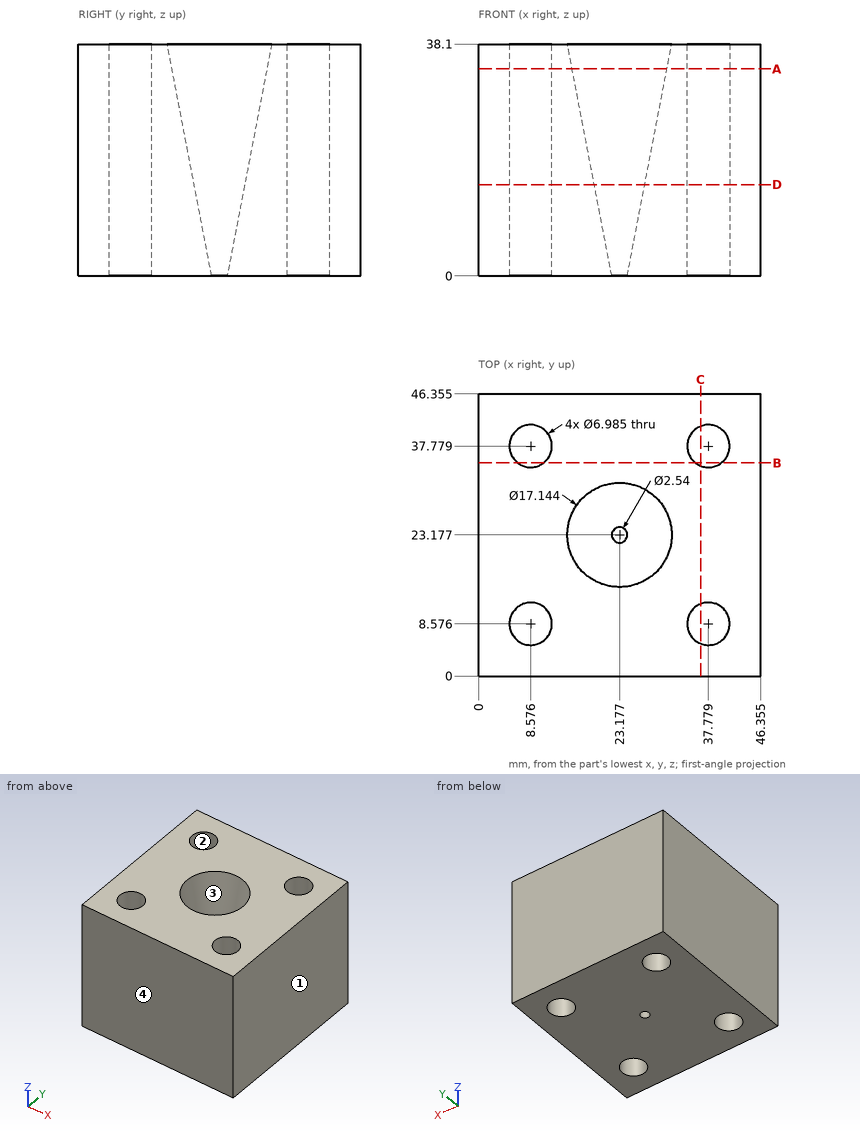
Here's the drawing with two shaded views (mm, measured from the low corner). I have some questions. Round coordinates to 2 decimals unless told otherwise and drop trailing zeros. Order: outer loops, then holes, each group sorted by start corner. A loop starts at its lowest first (then second) coordinate and runs counter-clockwise, first axis right, second up. Notation, with made-up numbers: (76.25, 32.5) -> (91.25, 32.5) arc R20 cw to (91.25, 57.5) -> close; hole circle Ø4 at (86.5, -15.5). An arc over 180 degrees is marked (long way). Use a Markdown table: item, result. Add a question column.
(1) Suppose I cut it at C-C, the plane x = 36.5. Please give me the cut outline in (y, z) (1 decimal), and give its area (3 significant figures).
(2) For pin 1 Ø5.5 at (x, y) = (37.78, 8.58) entering from -Z, with a flat end and sliding along its axis, tell me the tip position at first contact or that it passes through.
(3) Suppose I cut it at B-B, the plane y = 35. Please give me the cut outline in (x, z) (1 decimal), and give its area (3 significant figures).
(4) If we mould it in two halves opening along X, with no side actions, what happens to the marked faces 1, 2, 3 and 4? For each: released by +X, released by -X, zero draft, split by the parting line, or undercut.
(5) I need wall thicknesses on line 1 along Y through (x, z) = (37.5, 3) (1 decimal); line 2 along Y through (x, z) = (40, 33) (1 decimal). Which ranges of each line are inside material? Lowest first, please.
(6) Suppose I cut it at A-A, the plane z = 34. Please give me the cut outline in (x, y) (1 decimal), and give its area (4 significant figures).
(7) Suppose I cut it at D-D, the plane z = 15. Please give me the cut outline in (x, y) (1 decimal), and give its area (3 significant figures).
Verdict:
| question | item | result |
|---|---|---|
| 1 | outline | (0, 0) -> (5.3, 0) -> (5.3, 38.1) -> (0, 38.1) -> close; (11.8, 0) -> (34.5, 0) -> (34.5, 38.1) -> (11.8, 38.1) -> close; (41, 0) -> (46.4, 0) -> (46.4, 38.1) -> (41, 38.1) -> close |
| 1 | area | 1,270 mm2 |
| 2 | pin 1 | through |
| 3 | outline | (0, 0) -> (6.5, 0) -> (6.5, 38.1) -> (0, 38.1) -> close; (10.7, 0) -> (35.7, 0) -> (35.7, 38.1) -> (10.7, 38.1) -> close; (39.9, 0) -> (46.4, 0) -> (46.4, 38.1) -> (39.9, 38.1) -> close |
| 3 | area | 1,440 mm2 |
| 4 | face 1 | released by +X |
| 4 | face 2 | undercut |
| 4 | face 3 | undercut |
| 4 | face 4 | zero draft |
| 5 | line 1 | 0 to 5.1, 12.1 to 34.3, 41.3 to 46.4 |
| 5 | line 2 | 0 to 5.9, 11.3 to 35.1, 40.5 to 46.4 |
| 6 | outline | (0, 0) -> (46.4, 0) -> (46.4, 46.4) -> (0, 46.4) -> close; hole circle Ø7 at (8.6, 8.6); hole circle Ø7 at (8.6, 37.8); hole circle Ø15.6 at (23.2, 23.2); hole circle Ø7 at (37.8, 8.6); hole circle Ø7 at (37.8, 37.8) |
| 6 | area | 1,805 mm2 |
| 7 | outline | (0, 0) -> (46.4, 0) -> (46.4, 46.4) -> (0, 46.4) -> close; hole circle Ø7 at (8.6, 8.6); hole circle Ø7 at (8.6, 37.8); hole circle Ø8.3 at (23.2, 23.2); hole circle Ø7 at (37.8, 8.6); hole circle Ø7 at (37.8, 37.8) |
| 7 | area | 1,940 mm2 |
